Part print with two shaded views. Sizes in mm from the minimum x, y, z corner. A direction names the side the tool comes from. Coordinates: 2 decimals unless noted, no trailing zeros. Order: outer loops, then holes, each group sorted by start corner. A loop starts at its lowest first (then second) coordinate and runs counter-clockwise, first axis right, second up. Notation, with made-up numbers: (64, 76) - (118, 76) arc R14 cw to (118, 86) - close; hole circle Ø7 at (21.25, 54). An arc over 180 degrees is marked (long way). Return JSON: item names as keys, results as strings.
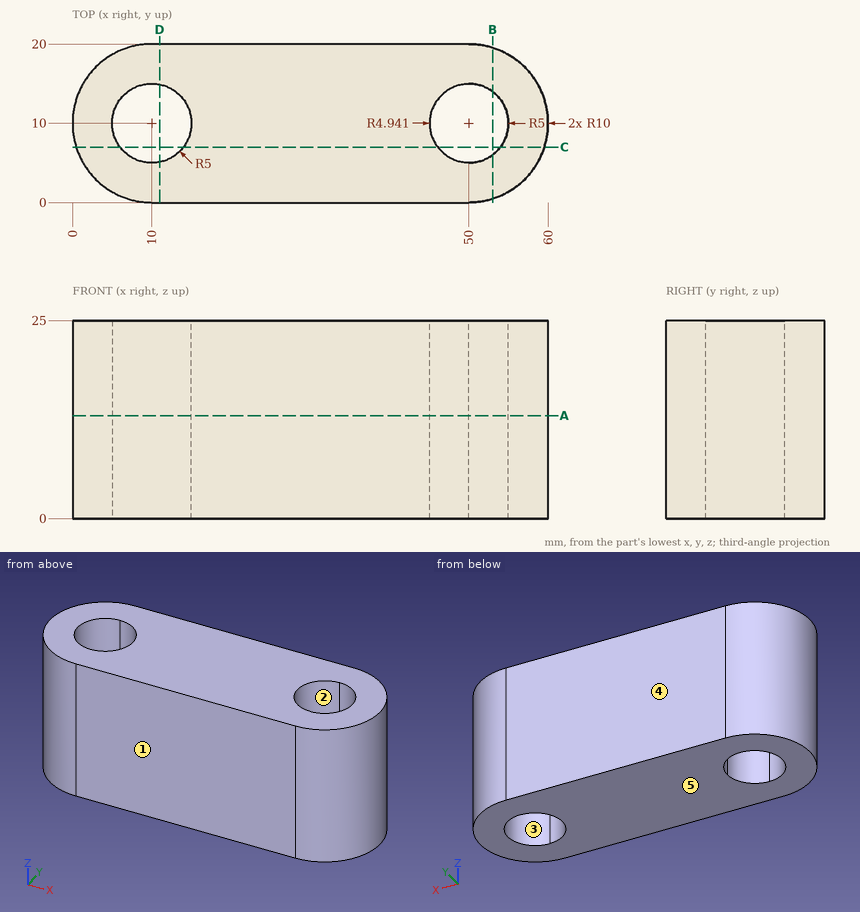
Item 1: Band-saw the part on A-A, the plane z = 13. List the corners of the cut face in (x, y).
Findings below:
{"outline": "(10, 0) - (50, 0) arc R10 ccw to (50, 20) - (10, 20) arc R10 ccw to start; hole circle Ø10 at (10, 10); hole (50, 5) arc R5 ccw to (50, 15) - (50, 14.94) arc R4.94 ccw to (50, 5.06) - close"}
Item 2: Drop flat-ended pins along their axis: P1, Ø5, axis at y = 3, z = 5, coming from the -X side; P2, Ø4, axis at y = 3, z = 11, coming from the +X side; P3, Ø6, axis at x = 9, y = 13, coming from the +Z side; P4, Ø1.5, axis at y = 9, z = 12.5, coming from the +X side. Give the stop position or say it passes through.
Findings below:
{"P1": "stops at x = 1.07", "P2": "stops at x = 58.66", "P3": "stops at z = 25", "P4": "stops at x = 60"}
Item 3: Which spindle directions (+Z, -Z, +X, -X, +Y, -Y) get a long thin tool onto all of the face, cutting with end or side? Do the marked faces 1 and 2. Say none if no direction does.
Findings below:
{"face 1": "+Z, -Z, +X, -X, -Y", "face 2": "+Z, -Z"}
Item 4: Wall check: L1, parallel to X at y = 12.25, z = 18 (1 decimal); L2, parallel to X at y = 13, z = 10.25; L3, parallel to X at y = 18.25, z = 5.75. Give the ranges that are in metal, low to high. Write a range as [from, to].
Findings below:
{"L1": "x = [0.3, 5.5], [14.5, 45.6], [54.5, 59.7]", "L2": "x = [0.46, 6], [14, 46.07], [54, 59.54]", "L3": "x = [4.35, 55.65]"}
Item 5: Band-saw the part on C-C, the plane y = 7. List the corners of the cut face in (x, z).
Findings below:
{"outline": "(0.46, 0) - (6, 0) - (6, 25) - (0.46, 25) - close; (14, 0) - (46.07, 0) - (46.07, 25) - (14, 25) - close; (54, 0) - (59.54, 0) - (59.54, 25) - (54, 25) - close"}
Item 6: Mould opens along Y. For the marked faces 3, 4 and 5 say: released by +Y, released by -Y, zero draft, split by the parting line, or undercut.
Findings below:
{"face 3": "undercut", "face 4": "released by +Y", "face 5": "zero draft"}
Item 7: Band-saw the part on B-B, the plane x = 53. List the corners of the cut face in (y, z), then the cut area to 3 significant figures.
Findings below:
{"outline": "(0.46, 0) - (6, 0) - (6, 25) - (0.46, 25) - close; (14, 0) - (19.54, 0) - (19.54, 25) - (14, 25) - close", "area": "277 mm²"}
Item 8: Band-saw the part on D-D, the plane x = 11. List the corners of the cut face in (y, z), then the cut area to 3 significant figures.
Findings below:
{"outline": "(0, 0) - (5.1, 0) - (5.1, 25) - (0, 25) - close; (14.9, 0) - (20, 0) - (20, 25) - (14.9, 25) - close", "area": "255 mm²"}
